Part model, mm, in its own coordinate system. A direction names the side the tool comes from. Give positions to 0.01 mm unless a question says otherwise; leave off trailing zeros. Loops run counter-clockwise (first coordinate to the right, second up) from the corner with the lowest first, then second, coordinate; pieces in that order, holes last. Notation, with made-up numbers: M -32,15 L -2,15 A18 ccw -2,46 Z; hole C 54,18.25 d3. An arc over 180 degrees is marked long. Put each result on its own line as item: value. Start each with the question number.
```python
from build123d import *

# Parameters (mm, degrees)
BOSS_EXTRUDE2_DEPTH = 10


with BuildPart() as part:
    # Sketch1 → Boss-Extrude2 (new body)
    with BuildSketch(Plane.XY):
        with BuildLine():
            Line((-49.595588235, 30.790441176), (-49.595588235, 55.790441176))
            Line((-49.595588235, 55.790441176), (-84.595588235, 55.790441176))
            Line((-84.595588235, 55.790441176), (-84.595588235, 5.790441176))
            Line((-84.595588235, 5.790441176), (-76.571127836, 5.790441176))
            Line((-76.571127836, 5.790441176), (-80.122995865, 8.369201143))
            Line((-80.122995865, 8.369201143), (-74.161024923, 10.431488509))
            ThreePointArc((-74.161024923, 10.431488509), (-65.548234046, 25.0391578), (-49.595588235, 30.790441176))
        make_face()
        with BuildLine():
            Line((10.404411765, 55.790441176), (-49.595588235, 55.790441176))
            Line((-49.595588235, 55.790441176), (-49.595588235, 30.790441176))
            ThreePointArc((-49.595588235, 30.790441176), (-46.420318597, 30.587974576), (-43.296479842, 29.983854194))
            Line((-43.296479842, 29.983854194), (-38.907655076, 38.5487403))
            Line((-38.907655076, 38.5487403), (-38.907655076, 28.390620042))
            ThreePointArc((-38.907655076, 28.390620042), (-30.648795615, 22.100531594), (-25.657089919, 12.997957973))
            Line((-25.657089919, 12.997957973), (-17.962154019, 12.997957973))
            Line((-17.962154019, 12.997957973), (-22.478851702, 5.790441176))
            Line((-22.478851702, 5.790441176), (-14.595588235, 5.790441176))
            ThreePointArc((-14.595588235, 5.790441176), (-12.499276658, 15.811471895), (-6.561903703, 24.151926396))
            Line((-6.561903703, 24.151926396), (-6.561903703, 35.084441479))
            Line((-6.561903703, 35.084441479), (0, 28.522537776))
            ThreePointArc((0, 28.522537776), (5.080053353, 30.216886016), (10.404411765, 30.790441176))
            Line((10.404411765, 30.790441176), (10.404411765, 55.790441176))
        make_face()
        with BuildLine():
            Line((70.404411765, 55.790441176), (10.404411765, 55.790441176))
            Line((10.404411765, 55.790441176), (10.404411765, 30.790441176))
            ThreePointArc((10.404411765, 30.790441176), (17.859813508, 29.652900917), (24.63674968, 26.343799964))
            Line((24.63674968, 26.343799964), (32.552494412, 30.790441176))
            Line((32.552494412, 30.790441176), (29.92126971, 21.41389329))
            ThreePointArc((29.92126971, 21.41389329), (33.993831518, 14.069286246), (35.404411765, 5.790441176))
            Line((35.404411765, 5.790441176), (45.404411765, 5.790441176))
            ThreePointArc((45.404411765, 5.790441176), (50.185133178, 20.493528384), (62.698873639, 29.573306483))
            Line((62.698873639, 29.573306483), (67.171172857, 38.5487403))
            Line((67.171172857, 38.5487403), (70.404411765, 30.790441176))
            Line((70.404411765, 30.790441176), (70.404411765, 55.790441176))
        make_face()
        with BuildLine():
            Line((130.404411765, 55.790441176), (70.404411765, 55.790441176))
            Line((70.404411765, 55.790441176), (70.404411765, 30.790441176))
            ThreePointArc((70.404411765, 30.790441176), (83.787720088, 26.906479118), (93.012607471, 16.461405843))
            Line((93.012607471, 16.461405843), (98.474145882, 18.660683713))
            Line((98.474145882, 18.660683713), (94.969848452, 10.431488509))
            ThreePointArc((94.969848452, 10.431488509), (95.295533849, 8.1211152), (95.404411765, 5.790441176))
            Line((95.404411765, 5.790441176), (105.404411765, 5.790441176))
            ThreePointArc((105.404411765, 5.790441176), (106.107781477, 11.678883811), (108.178312298, 17.23598627))
            Line((108.178312298, 17.23598627), (105.404411765, 23.549684511))
            Line((105.404411765, 23.549684511), (110.88755382, 21.41389329))
            ThreePointArc((110.88755382, 21.41389329), (119.578200582, 28.324707338), (130.404411765, 30.790441176))
            Line((130.404411765, 30.790441176), (130.404411765, 55.790441176))
        make_face()
        with BuildLine():
            Line((165.404411765, 55.790441176), (130.404411765, 55.790441176))
            Line((130.404411765, 55.790441176), (130.404411765, 30.790441176))
            ThreePointArc((130.404411765, 30.790441176), (133.401752606, 30.610109746), (136.355852267, 30.071717007))
            Line((136.355852267, 30.071717007), (140.818257218, 36.687543597))
            Line((140.818257218, 36.687543597), (142.579811014, 27.625267787))
            ThreePointArc((142.579811014, 27.625267787), (151.961139035, 18.451701358), (155.404411765, 5.790441176))
            Line((155.404411765, 5.790441176), (165.404411765, 5.790441176))
            Line((165.404411765, 5.790441176), (165.404411765, 55.790441176))
        make_face()
        with BuildLine():
            Line((165.404411765, -44.209558824), (165.404411765, 5.790441176))
            Line((165.404411765, 5.790441176), (155.404411765, 5.790441176))
            ThreePointArc((155.404411765, 5.790441176), (151.961139035, -6.870819005), (142.579811014, -16.044385434))
            Line((142.579811014, -16.044385434), (139.723435627, -21.807209952))
            Line((139.723435627, -21.807209952), (132.176529952, -19.14667167))
            ThreePointArc((132.176529952, -19.14667167), (131.291028602, -19.193832089), (130.404411765, -19.209558824))
            Line((130.404411765, -19.209558824), (130.404411765, -44.209558824))
            Line((130.404411765, -44.209558824), (165.404411765, -44.209558824))
        make_face()
        with BuildLine():
            ThreePointArc((78.603951233, -17.826661789), (74.562080934, -18.861410419), (70.404411765, -19.209558824))
            Line((70.404411765, -19.209558824), (70.404411765, -44.209558824))
            Line((70.404411765, -44.209558824), (130.404411765, -44.209558824))
            Line((130.404411765, -44.209558824), (130.404411765, -19.209558824))
            ThreePointArc((130.404411765, -19.209558824), (124.758153779, -18.563609221), (119.403671642, -16.659140484))
            Line((119.403671642, -16.659140484), (108.178312298, -21.807209952))
            Line((108.178312298, -21.807209952), (110.88755382, -9.833010937))
            ThreePointArc((110.88755382, -9.833010937), (106.814992011, -2.488403893), (105.404411765, 5.790441176))
            Line((105.404411765, 5.790441176), (95.404411765, 5.790441176))
            ThreePointArc((95.404411765, 5.790441176), (92.88136777, -5.154258396), (85.821495865, -13.889841287))
            Line((85.821495865, -13.889841287), (89.988841167, -19.209558824))
            Line((89.988841167, -19.209558824), (78.603951233, -17.826661789))
        make_face()
        with BuildLine():
            ThreePointArc((16.26584722, -18.512718585), (13.35576789, -19.034737514), (10.404411765, -19.209558824))
            Line((10.404411765, -19.209558824), (10.404411765, -44.209558824))
            Line((10.404411765, -44.209558824), (70.404411765, -44.209558824))
            Line((70.404411765, -44.209558824), (70.404411765, -19.209558824))
            ThreePointArc((70.404411765, -19.209558824), (66.503875434, -18.903400492), (62.698873639, -17.99242413))
            Line((62.698873639, -17.99242413), (57.774840306, -22.916457463))
            Line((57.774840306, -22.916457463), (57.774840306, -15.784867043))
            ThreePointArc((57.774840306, -15.784867043), (48.716404866, -6.644604331), (45.404411765, 5.790441176))
            Line((45.404411765, 5.790441176), (35.404411765, 5.790441176))
            ThreePointArc((35.404411765, 5.790441176), (32.092418663, -6.644604331), (23.033983223, -15.784867043))
            Line((23.033983223, -15.784867043), (24.63674968, -26.883621045))
            Line((24.63674968, -26.883621045), (16.26584722, -18.512718585))
        make_face()
        with BuildLine():
            ThreePointArc((-24.894580949, 1.935543121), (-33.337858557, -13.20129981), (-49.595588235, -19.209558824))
            Line((-49.595588235, -19.209558824), (-49.595588235, -44.209558824))
            Line((-49.595588235, -44.209558824), (10.404411765, -44.209558824))
            Line((10.404411765, -44.209558824), (10.404411765, -19.209558824))
            ThreePointArc((10.404411765, -19.209558824), (0.386918535, -17.114794674), (-7.951831841, -11.181545175))
            Line((-7.951831841, -11.181545175), (-15.042390882, -13.889841287))
            Line((-15.042390882, -13.889841287), (-11.571398063, -6.128610062))
            ThreePointArc((-11.571398063, -6.128610062), (-13.827749155, -0.357922603), (-14.595588235, 5.790441176))
            Line((-14.595588235, 5.790441176), (-22.478851702, 5.790441176))
            Line((-22.478851702, 5.790441176), (-24.894580949, 1.935543121))
        make_face()
        with BuildLine():
            Line((-76.571127836, 5.790441176), (-84.595588235, 5.790441176))
            Line((-84.595588235, 5.790441176), (-84.595588235, -44.209558824))
            Line((-84.595588235, -44.209558824), (-49.595588235, -44.209558824))
            Line((-49.595588235, -44.209558824), (-49.595588235, -19.209558824))
            ThreePointArc((-49.595588235, -19.209558824), (-55.612209406, -18.474765802), (-61.275152877, -16.313580398))
            Line((-61.275152877, -16.313580398), (-69.988075999, -18.512718585))
            Line((-69.988075999, -18.512718585), (-67.951831841, -11.181545175))
            ThreePointArc((-67.951831841, -11.181545175), (-72.598243173, -4.001283177), (-74.552596729, 4.324928615))
            Line((-74.552596729, 4.324928615), (-76.571127836, 5.790441176))
        make_face()
    extrude(amount=BOSS_EXTRUDE2_DEPTH)


solid = part.part
```
1) Mould opens along Y. For faces 3 (the flat face through (136.003, -20.496, 4.93)), 4 (the flat face through (42, 55.79, 5)), 5 (the flat face through (39, 6, 0)) say: +Y half, -Y half, draft (parallel to the pull), parting line (faces both ways), or undercut.
2) Wall check: L1, parallel to Y at x = 72, z = 8; L2, parallel to X at y = 36.5, z = 9.75; L3, parallel to X at y = 31, z = 9.5. Give the ranges that are in metal, low to high.
3) Which spindle directions (+Z, -Z, +X, -X, +Y, -Y) get a long thin tool onto all of the face, cutting with end or side? Do faces 1 (the flat face through (141.17, -18.89, 4.93)), 2 (the flat face through (39, -44.21, 5)). Say none if no direction does.
4) Band-saw the part on A-A on x = -45.5. Give the cut face in (y, z).
5) Band-saw the part on C-C on x = 3. Give the cut face in (y, z).
6) Band-saw the part on B-B on z = 1.5. State how many separate pieces and enclosed holes the cut face has, then the cut area to 3 significant figures.
7) Pin check, flat tip, straight feed: pin 1 Ø12 at (x, y) = (99.5, -1) entering from -Z. Stop position of the tip, or through.
Evaluation:
1. face 3: undercut
1. face 4: +Y half
1. face 5: draft
2. L1: -44.21 to -19.16, 30.74 to 55.79
2. L2: -84.6 to -39.96, -38.91 to 66.15, 68.02 to 140.69, 140.85 to 165.4
2. L3: -84.6 to -42.78, -38.91 to -6.56, -2.48 to 63.41, 70.32 to 136.98, 141.92 to 165.4
3. face 1: +Z, -Z
3. face 2: +Z, -Z, +X, -X, -Y
4. outline: M -44.21,0 L -18.87,0 L -18.87,10 L -44.21,10 Z; M 30.45,0 L 55.79,0 L 55.79,10 L 30.45,10 Z
5. outline: M -44.21,0 L -18.09,0 L -18.09,10 L -44.21,10 Z; M 29.67,0 L 55.79,0 L 55.79,10 L 29.67,10 Z
6. separate pieces: 1
6. enclosed holes: 4
6. area: 16,700 mm2
7. pin 1: z = 0
